Here's how the part is built. I have some questions about the finished solid (model axes, mm). A direction names the side the tool comes from. Round coordinates to 2 decimals unless told otherwise and drop trailing zeros. Write each loop counter-clockwise with the first axis right and the second up, starting at its lowest first coordinate (ties: lowest second). Pieces come first, ordered by that corner, then holes. Notation, with made-up numbers: (28, 79) -> (65, 79) arc R26 cw to (65, 116) -> close; hole circle Ø8 at (-13.75, 27). An arc over 180 degrees is marked (long way). Put each result on its own line as item: value. Start each with the question number.
1) Which directions (+Z, -Z, +X, -X, +Y, -Y) give clear straight access to the entire face, cutting with the end or side of a thin tool? Please do faces 1 (the flat face through (4, 3.4, 0)), 2 (the cylindrical face through (1.08, -4.88, -9.86)), 3 (the flat face through (-5, -30, 2)).
2) I want a section at B-B, the plane x = 0. List the corners of the cut face in (y, z) for me, then the cut area to 3 significant figures.
3) If I drill on line 1 along X through (y, z) = (-12, 3); line 2 along Z through (x, y) = (0, -40); line 3 along Y through (x, z) = (-19.5, 1.75), over which ranges is the centre line in solid material (lowest first)? Write a range as [from, to].
4) Will these pins go through, and if not, where does the flat tip stop? P1, Ø10, axis at x = -31.5, z = -1, coming from the -Y side; P2, Ø5.5, axis at y = -21.5, z = 2.5, coming from the -X side; P3, Ø3, axis at y = 5.5, z = -14, coming from the +X side.
5) I want a section at D-D, the plane z = -13.75. List the corners of the cut face in (x, y) for me, then the cut area to 3 significant figures.
6) I want a section at C-C, the plane y = -44. List the corners of the cut face in (x, z) for me.
7) I want a section at A-A, the plane z = 3. List the corners of the cut face in (x, y) for me.
from build123d import *

# Parameters (mm, degrees)
BOSS_EXTRU_1_DEPTH = 5
ESQUISSE2_R        = 5
BOSS_EXTRU_2_DEPTH = 20


with BuildPart() as part:
    # Esquisse1 → Boss.-Extru.1 (new body)
    with BuildSketch(Plane.XY):
        Polygon((5, -5.958767963), (-5, -4.195498156), (-5, -55.804501844), (5, -55.804501844), align=None)
        Polygon((-52.351983404, 14.308200227), (-54.088465181, 4.460122697), (-5, -4.195498156), (5, -5.958767963), (5, 4.195498156), align=None)
    extrude(amount=BOSS_EXTRU_1_DEPTH)

    # Esquisse2 → Boss.-Extru.2 (add)
    with BuildSketch(Plane(origin=(0, 0, 0), x_dir=(-1, 0, 0), z_dir=(0, 0, -1))):
        Circle(ESQUISSE2_R)
    extrude(amount=BOSS_EXTRU_2_DEPTH)


solid = part.part
Findings:
1. face 1: -Z, +X, +Y
1. face 2: -Z
1. face 3: +Z, -Z, -X, -Y
2. outline: (-55.8, 0) -> (-5, 0) -> (-5, -20) -> (5, -20) -> (5, 0) -> (5.08, 0) -> (5.08, 5) -> (-55.8, 5) -> close
2. area: 504 mm2
3. line 1: x = [-5, 5]
3. line 2: z = [0, 5]
3. line 3: y = [-1.64, 8.52]
4. P1: stops at y = -0.39
4. P2: stops at x = -5
4. P3: stops at x = 3
5. outline: circle Ø10 at (0, 0)
5. area: 78.5 mm2
6. outline: (-5, 0) -> (5, 0) -> (5, 5) -> (-5, 5) -> close
7. outline: (-54.09, 4.46) -> (-5, -4.2) -> (-5, -55.8) -> (5, -55.8) -> (5, 4.2) -> (-52.35, 14.31) -> close
